Work out the finished part from the listing and answer in its coordinate system (mm). Coordinates: 2 decimals unless noted, no trailing zeros. One line per item, written item: value.
```python
from build123d import *

# Parameters (mm, degrees)
SKETCH_1_W          = 96.4
SKETCH_1_H          = 83.2
SKETCH_1_R          = 1.6
EXTRUDE_1_DEPTH     = 3
FILLET_1_R          = 2
CUT_EXTRUDE_3_DEPTH = 3


with BuildPart() as part:
    # Sketch 1 → Extrude 1 (new body)
    with BuildSketch(Plane.XY):
        Rectangle(SKETCH_1_W, SKETCH_1_H)
        with Locations((45.2, 38.6)):
            Circle(SKETCH_1_R, mode=Mode.SUBTRACT)
        with Locations((45.2, -38.6)):
            Circle(SKETCH_1_R, mode=Mode.SUBTRACT)
        with Locations((-45.2, 38.6)):
            Circle(SKETCH_1_R, mode=Mode.SUBTRACT)
        with Locations((-45.2, -38.6)):
            Circle(SKETCH_1_R, mode=Mode.SUBTRACT)
    extrude(amount=EXTRUDE_1_DEPTH)

    # Fillet 1
    fillet_1_edges = [part.edges().sort_by_distance(p)[0] for p in [
        (48.2, -41.6, 1.5),
        (-48.2, -41.6, 1.5),
        (-48.2, 41.6, 1.5),
        (48.2, 41.6, 1.5),
    ]]
    fillet(fillet_1_edges, radius=FILLET_1_R)

    # Sketch 1_3 → Cut-Extrude 3 (cut)
    with BuildSketch(Plane.XY):
        with BuildLine():
            ThreePointArc((41.7, 33.6), (40.2, 35.1), (38.7, 33.6))
            Line((38.7, 33.6), (40.2, 33.6))
            Line((40.2, 33.6), (40.2, 32.1))
            ThreePointArc((40.2, 32.1), (41.260660172, 32.539339828), (41.7, 33.6))
        make_face()
        with BuildLine():
            Line((40.2, 33.6), (38.7, 33.6))
            ThreePointArc((38.7, 33.6), (39.139339828, 32.539339828), (40.2, 32.1))
            Line((40.2, 32.1), (40.2, 33.6))
        make_face()
        with BuildLine():
            ThreePointArc((41.7, 33.6), (40.2, 35.1), (38.7, 33.6))
            Line((38.7, 33.6), (40.2, 33.6))
            Line((40.2, 33.6), (40.2, 32.1))
            ThreePointArc((40.2, 32.1), (41.260660172, 32.539339828), (41.7, 33.6))
        make_face()
        with BuildLine():
            Line((40.2, 33.6), (38.7, 33.6))
            ThreePointArc((38.7, 33.6), (39.139339828, 32.539339828), (40.2, 32.1))
            Line((40.2, 32.1), (40.2, 33.6))
        make_face()
        with BuildLine():
            ThreePointArc((41.7, -33.6), (41.260660172, -32.539339828), (40.2, -32.1))
            Line((40.2, -32.1), (40.2, -33.6))
            Line((40.2, -33.6), (38.7, -33.6))
            ThreePointArc((38.7, -33.6), (40.2, -35.1), (41.7, -33.6))
        make_face()
        with BuildLine():
            Line((40.2, -33.6), (40.2, -32.1))
            ThreePointArc((40.2, -32.1), (39.139339828, -32.539339828), (38.7, -33.6))
            Line((38.7, -33.6), (40.2, -33.6))
        make_face()
        with BuildLine():
            ThreePointArc((41.7, -33.6), (41.260660172, -32.539339828), (40.2, -32.1))
            Line((40.2, -32.1), (40.2, -33.6))
            Line((40.2, -33.6), (38.7, -33.6))
            ThreePointArc((38.7, -33.6), (40.2, -35.1), (41.7, -33.6))
        make_face()
        with BuildLine():
            Line((40.2, -33.6), (40.2, -32.1))
            ThreePointArc((40.2, -32.1), (39.139339828, -32.539339828), (38.7, -33.6))
            Line((38.7, -33.6), (40.2, -33.6))
        make_face()
        with BuildLine():
            ThreePointArc((-38.7, -33.6), (-39.139339828, -32.539339828), (-40.2, -32.1))
            Line((-40.2, -32.1), (-40.2, -33.6))
            Line((-40.2, -33.6), (-38.7, -33.6))
        make_face()
        with BuildLine():
            Line((-40.2, -33.6), (-40.2, -32.1))
            ThreePointArc((-40.2, -32.1), (-41.260660172, -34.660660172), (-38.7, -33.6))
            Line((-38.7, -33.6), (-40.2, -33.6))
        make_face()
        with BuildLine():
            ThreePointArc((-38.7, -33.6), (-39.139339828, -32.539339828), (-40.2, -32.1))
            Line((-40.2, -32.1), (-40.2, -33.6))
            Line((-40.2, -33.6), (-38.7, -33.6))
        make_face()
        with BuildLine():
            Line((-40.2, -33.6), (-40.2, -32.1))
            ThreePointArc((-40.2, -32.1), (-41.260660172, -34.660660172), (-38.7, -33.6))
            Line((-38.7, -33.6), (-40.2, -33.6))
        make_face()
        with BuildLine():
            ThreePointArc((-40.2, 32.1), (-39.139339828, 32.539339828), (-38.7, 33.6))
            Line((-38.7, 33.6), (-40.2, 33.6))
            Line((-40.2, 33.6), (-40.2, 32.1))
        make_face()
        with BuildLine():
            Line((-40.2, 33.6), (-38.7, 33.6))
            ThreePointArc((-38.7, 33.6), (-41.260660172, 34.660660172), (-40.2, 32.1))
            Line((-40.2, 32.1), (-40.2, 33.6))
        make_face()
        with BuildLine():
            ThreePointArc((-40.2, 32.1), (-39.139339828, 32.539339828), (-38.7, 33.6))
            Line((-38.7, 33.6), (-40.2, 33.6))
            Line((-40.2, 33.6), (-40.2, 32.1))
        make_face()
        with BuildLine():
            Line((-40.2, 33.6), (-38.7, 33.6))
            ThreePointArc((-38.7, 33.6), (-41.260660172, 34.660660172), (-40.2, 32.1))
            Line((-40.2, 32.1), (-40.2, 33.6))
        make_face()
    extrude(amount=CUT_EXTRUDE_3_DEPTH, mode=Mode.SUBTRACT)


solid = part.part
```
Item 1: Given pin 1 (4 mm diameter, centred on x = -40.2, y = -33.6, fed in from +Z); pin 2 (2.5 mm diameter, centred on x = 45.2, y = -38.6, fed in from +Z), each flat-ended and moving along its own axis, determine where each tip first touches the part or whether it passes through.
Evaluation:
pin 1: stops at z = 3
pin 2: passes through
Item 2: Determine the mould class of faces 1 (the face through (-44.34, 39.95, 1.48)), 2 (the face through (-1, 1, 3)), 3 (the face through (-1, 41.6, 1)), 4 (the face through (-1, -41.6, 1)) for opening direction Y: +Y half, -Y half, draft (parallel to the pull), parting line (faces both ways), or undercut.
Evaluation:
face 1: undercut
face 2: draft
face 3: +Y half
face 4: -Y half
Item 3: Consider probe 1 along Y at (x, z) = (45.2, 1.1); probe 2 along X at (y, z) = (33.6, 1.1); probe 3 along Y at (x, z) = (-40.2, 1.4). Determine where each line is inside the solid, lowest interval first.
Evaluation:
probe 1: y = -41.6 to -40.2, -37 to 37, 40.2 to 41.6
probe 2: x = -48.2 to -41.7, -38.7 to 38.7, 41.7 to 48.2
probe 3: y = -41.6 to -35.1, -32.1 to 32.1, 35.1 to 41.6
